Source: CAD feature listing. Evaluate the final solid. Frame: model axes, mm. Face numbers are marked on the shaded views. Round coordinates to 2 decimals unless told otherwise and drop trailing zeros. Order: outer loops, then holes, each group sorted by start corner. A loop starts at its lowest first (then second) coordinate and runs counter-clockwise, first axis right, second up. Notation, with made-up numbers: (-19, -39) -> (31, -39) arc R15 cw to (31, -12) -> close; hole circle Ø1 at (65, 61). An arc over 180 degrees is marked (long way). One line per item, written item: value. Start each with the question number.
1) Section D-D (y = 8.25). Return the cut outline in (x, z), and give its area (3 significant figures).
2) Section C-C (x = 0). Return the cut outline in (y, z).
3) Mould query, pull axis Y, two halves, no side actions, for the marked faces 1, 2 and 3. Classes: pulls with the +Y half, pulls with the -Y half, needs draft (parallel to the pull), parting line crosses it, or undercut.
4) Section A-A (y = 3). Return the cut outline in (x, z), and give its area (3 significant figures).
5) Section B-B (z = 3.75). Return the cut outline in (x, y).
6) Ray query, L1, parallel to Y at x = 0, z = 7.25; L2, parallel to X at y = 4.25, z = 8; L3, parallel to Y at x = -4.25, z = 1. Return the intervals inside material, ascending.
7) Pin query (flat end, axial travel): P1, Ø1.5, axis at x = -1, y = 8.5, coming from the +Z side. Return the tip coordinate at first contact, or that it passes through.
```python
from build123d import *

# Parameters (mm, degrees)
SKETCH1_R           = 1.6
BOSS_EXTRUDE1_DEPTH = 10


with BuildPart() as part:
    # Sketch1 → Boss-Extrude1 (new body)
    with BuildSketch(Plane.XY):
        Polygon((7.5, 0), (-7.5, 0), (-7.5, 6), (-7.5, 6.78663835), (-2.068965517, 12), (2.068965517, 12), (7.5, 6.78663835), (7.5, 6), align=None)
        with Locations((0, 9)):
            Circle(SKETCH1_R, mode=Mode.SUBTRACT)
        with Locations((-4.5, 3)):
            Circle(SKETCH1_R, mode=Mode.SUBTRACT)
        with Locations(Location((4.5, 3, 0), (0, 0, 180))):
            Circle(SKETCH1_R, mode=Mode.SUBTRACT)
    extrude(amount=BOSS_EXTRUDE1_DEPTH)


solid = part.part
```
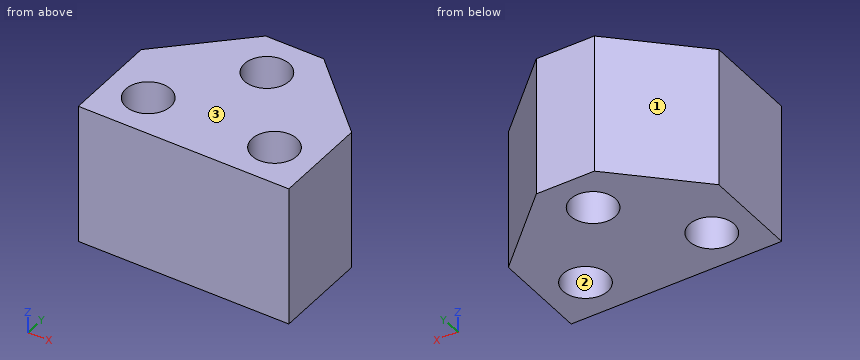
Findings:
1. outline: (-5.98, 0) -> (-1.41, 0) -> (-1.41, 10) -> (-5.98, 10) -> close; (1.41, 0) -> (5.98, 0) -> (5.98, 10) -> (1.41, 10) -> close
1. area: 91.2 mm2
2. outline: (0, 0) -> (7.4, 0) -> (7.4, 10) -> (0, 10) -> close; (10.6, 0) -> (12, 0) -> (12, 10) -> (10.6, 10) -> close
3. face 1: pulls with the +Y half
3. face 2: undercut
3. face 3: needs draft
4. outline: (-7.5, 0) -> (-6.1, 0) -> (-6.1, 10) -> (-7.5, 10) -> close; (-2.9, 0) -> (2.9, 0) -> (2.9, 10) -> (-2.9, 10) -> close; (6.1, 0) -> (7.5, 0) -> (7.5, 10) -> (6.1, 10) -> close
4. area: 86.0 mm2
5. outline: (-7.5, 0) -> (7.5, 0) -> (7.5, 6.79) -> (2.07, 12) -> (-2.07, 12) -> (-7.5, 6.79) -> close; hole circle Ø3.2 at (-4.5, 3); hole circle Ø3.2 at (0, 9); hole circle Ø3.2 at (4.5, 3)
6. L1: 0 to 7.4, 10.6 to 12
6. L2: -7.5 to -5.5, -3.5 to 3.5, 5.5 to 7.5
6. L3: 0 to 1.42, 4.58 to 9.91
7. P1: z = 10
